For this review, take the finished solid that the model builds, in its own axes (mm). A direction names the side the tool comes from. Coordinates: 2 decimals unless noted, no trailing zeros. Loops run counter-clockwise (first coordinate to the right, second up) from the corner with the lowest first, then second, coordinate; pieces in that order, holes last. Notation, with made-up numbers: (84.25, 54) -> (123.25, 54) arc R17 ccw to (123.25, 59) -> close; hole circle Ø1 at (54.5, 31). An arc over 180 degrees is marked (long way). One line per item, written item: value.
from build123d import *

# Parameters (mm, degrees)
F0_W        = 22.5
F0_H        = 15
F0_R        = 17.5
F1_DEPTH    = 60
F2_R        = 10
F3_DEPTH    = 75.9
F4_T1_DEPTH = 407.2453152316
F5_R        = 34.99999


# Not quite as in the source:
# - a fillet or chamfer that OpenCascade refuses, or shapes differently, is made with other operations: its cross-section is extruded or revolved along the edge and cut away or added
# - a fillet or chamfer is up to 0.001 mm smaller than in the source, because OpenCascade refuses the exact size


with BuildPart() as f1:
    # F0 (on Front) → F1 (new body)
    with BuildSketch(Plane.XZ):
        Polygon((-24.4408938289, -40.7930500805), (10.5591061711, -40.7930500805), (13.0723165348, -40.7930500805), (45.5591061711, -40.7930500805), (45.5591061711, -35.7930500805), (-24.4408938289, -35.7930500805), align=None)
        Polygon((13.0723165348, -40.7930500805), (10.5591061711, -40.7930500805), (-24.4408938289, -40.7930500805), (-46.9408938289, -40.7930500805), (-46.9408938289, -55.7930500805), (68.0591061711, -55.7930500805), (68.0591061711, -40.7930500805), (45.5591061711, -40.7930500805), align=None)
        with Locations((-58.1908938289, -48.2930500805)):
            Rectangle(F0_W, F0_H)
        Polygon((-24.4408938289, 9.2069499195), (-24.4408938289, -35.7930500805), (45.5591061711, -35.7930500805), (45.5591061711, 9.2069499195), (45.5591061711, 34.2069499195), (-24.4408938289, 34.2069499195), align=None)
        with Locations((10.5591061711, 9.2069499195)):
            Circle(F0_R, mode=Mode.SUBTRACT)
        with Locations((79.3091061711, -48.2930500805)):
            Rectangle(F0_W, F0_H)
    extrude(amount=F1_DEPTH)

    # F2 (on Top) → F3 (cut)
    with BuildSketch(Plane.XY):
        with Locations((-46.9408938289, -30)):
            Circle(F2_R)
        with Locations((68.0591061711, -30)):
            Circle(F2_R)
    extrude(amount=-F3_DEPTH, mode=Mode.SUBTRACT)

    # F4: chamfer of 65 x 23.6580652273 on 1 edges, made by hand

    # F4_s2 → F4_t1 (cut)
    with BuildSketch(Plane.YZ.offset(-193.0635514447)):
        Polygon((-60, -30.7930500805), (-36.3419347727, 34.2069499195), (-60, 34.2069499195), align=None)
    extrude(amount=F4_T1_DEPTH, mode=Mode.SUBTRACT)

    # F5 (radius 35 in the source; OpenCascade refuses exactly that, so slightly less here)
    f5_edges = [f1.edges().sort_by_distance(p)[0] for p in [
        (45.559106, -18.170967, 34.20695),
        (-24.440894, -18.170967, 34.20695),
    ]]
    fillet(f5_edges, radius=F5_R)


solid = f1.part
1. Insertion check: pin 1 Ø6 at (x, y) = (-3.5, -38.5) entering from +Z; pin 2 Ø1 at (x, z) = (28.5, -46.5) entering from +Y; pin 3 Ø12 at (y, z) = (-21.5, -24.5) entering from +X; pin 4 Ø4 at (x, y) = (6, -43.5) entering from +Z. Each pin has a flat end and moves straight along its axis. Give the tip position at first contact, or say it passes through.
Return value:
pin 1: stops at z = 32.29
pin 2: stops at y = 0
pin 3: stops at x = 45.56
pin 4: stops at z = -7.02
2. Take a section at C-C, the plane x = 23.5. Give the boundary of the cut face in (y, z), and give its area (3 significant figures).
Return value:
outline: (-60, -55.79) -> (0, -55.79) -> (0, -2.57) -> (-49.73, -2.57) -> (-60, -30.79) -> close; (-41.15, 20.99) -> (0, 20.99) -> (0, 31.73) -> (-37.24, 31.73) -> close
area: 3,470 mm2
3. For faces 1 (the flat face through (-36.6, -29.6, -40.793)), 2 (the cylindrical face through (-42.327, -38.872, -48.188)), 3 (the flat face through (45.559, -30, -21)), list the 3-axis set-ups (+Z, -Z, +X, -X, +Y, -Y) from which the entire face can be reached by the end or side of a thin tool; tool diameter is ignored.
Return value:
face 1: +Z, -X, +Y, -Y
face 2: +Z, -Z
face 3: +Z, +X, +Y, -Y
4. Take a section at B-B, the plane z = -50. Give the boundary of the cut face in (x, y), and give its area (3 significant figures).
Return value:
outline: (-69.44, -60) -> (90.56, -60) -> (90.56, 0) -> (-69.44, 0) -> close; hole circle Ø20 at (-46.94, -30); hole circle Ø20 at (68.06, -30)
area: 8,970 mm2
5. The part is to be moulded in two halves that separate along X. For faces 4 (the cylindrical face through (72.673, -38.872, -48.188)), 5 (the flat face through (9, -30, -55.793)), 6 (the flat face through (90.559, -30, -48)), say which applies: pulls with the +X half, pulls with the -X half, needs draft (parallel to the pull), parting line crosses it, or undercut.
Return value:
face 4: undercut
face 5: needs draft
face 6: pulls with the +X half
6. Take a section at A-A, the plane y = -23. Give the number of separate pieces and of enclosed holes in the cut face, and give its area (3 significant figures).
Return value:
separate pieces: 3
enclosed holes: 1
area: 5,730 mm2
7. To check wall thickness, follow probe 1 along X at (y, z) = (-39, -49); probe 2 along X at (y, z) = (-31, -51); probe 3 along Z at (x, y) = (62, -50). State the ranges of each line that lie inside material, in increasing order. Write a range as from..to.
Return value:
probe 1: x = -69.44..-51.3, -42.58..63.7, 72.42..90.56
probe 2: x = -69.44..-56.89, -36.99..58.11, 78.01..90.56
probe 3: z = -55.79..-40.79
